Verification items for the finished model (mm, model axes). A direction names the side the tool comes from. Coordinates: 2 decimals unless noted, no trailing zeros. Write each loop counter-clockwise with the first axis right and the second up, starting at its lowest first coordinate (ties: lowest second). Pieces come first, ordered by that corner, then holes. Notation, with made-up numbers: (18, -17.75) -> (54, -17.75) arc R23 cw to (54, -4.75) -> close; hole circle Ø6 at (-14.75, 89.25). An arc over 180 degrees is marked (long way). Use CSV: the item, a comma, the result in double quotes.
```python
from build123d import *

# Parameters (mm, degrees)
F0_R            = 35.76066
F1_DEPTH        = 7.2136
F3_DEPTH        = 7.2146
F3_COPIES_COUNT = 16


# Not quite as in the source:
# - a pattern or mirror of a feature is missing from the dataset's text; its kind, count and spacing are read off the source's solid


with BuildPart() as f1:
    # F0 (on Front) → F1 (new body)
    with BuildSketch(Plane.XZ):
        Circle(F0_R)
    extrude(amount=-F1_DEPTH)

    # F2 (on face) → F3 (cut, through all)
    with BuildSketch(Plane.XZ):
        with BuildLine():
            Line((-4.8164154778, 33.0982711732), (-4.4568878106, 32.3001493474))
            ThreePointArc((-4.4568878106, 32.3001493474), (-3.8441959519, 31.1417538349), (-3.0902142758, 30.0699408338))
            ThreePointArc((-3.0902142758, 30.0699408338), (0, 28.5877), (3.0902142758, 30.0699408338))
            ThreePointArc((3.0902142758, 30.0699408338), (3.8441959519, 31.1417538349), (4.4568878106, 32.3001493474))
            Line((4.4568878106, 32.3001493474), (4.8164154778, 33.0982711732))
            ThreePointArc((4.8164154778, 33.0982711732), (5.4627291736, 34.2224644474), (6.3166306588, 35.198366166))
            ThreePointArc((6.3166306588, 35.198366166), (0, 35.76066), (-6.3166306588, 35.198366166))
            ThreePointArc((-6.3166306588, 35.198366166), (-5.4627291736, 34.2224644474), (-4.8164154778, 33.0982711732))
        make_face()
    f3 = extrude(amount=-F3_DEPTH, mode=Mode.SUBTRACT)

    # F3_copies: F3 ×16 about axis
    f3_copies_axis = Axis((0, 0, 0), (0, 1, 0))
    for i in range(1, F3_COPIES_COUNT):
        add(f3.rotate(f3_copies_axis, i * 360 / F3_COPIES_COUNT), mode=Mode.SUBTRACT)


solid = f1.part
```
1) Set-up check for faces 1 (the cylindrical face through (-18.1, 3.6, -29.5)), 2 (the cylindrical face through (-20.34, 3.56, -28.08)), 3 (the cylindrical face through (15.454, 3.556, 27.289)), 4 (the cylindrical face through (-33.726, 3.556, 8.045)), 5 (the cylindrical face through (34.237, 3.556, 5.473)): record each of +Z, -Z, +X, -X, +Y, -Y from which the full face is reachable in a straight line by a thin tool's end or side.
Return value:
face 1,"-Z, +Y, -Y"
face 2,"-X, +Y, -Y"
face 3,"+Z, +Y, -Y"
face 4,"+Z, -X, +Y, -Y"
face 5,"+X, +Y, -Y"
2) Scan lines: L1, parallel to X at y = 6.25, z = -28; L2, parallel to X at y = 4.25, z = 30; L3, parallel to Z at x = -27, y = 2.25. Record each from-to range of solid material in increasing order.
Return value:
L1,"-20.33 to -16.33, -9.08 to 9.08, 16.33 to 20.33"
L2,"-19.46 to -19.05, -8.41 to -3.03, 3.03 to 8.41, 19.05 to 19.46"
L3,"-20.07 to -15.03, -9.95 to 9.95, 15.03 to 20.07"
3) Cross-section at B-B (x = -10). Record the boundary of the cut face in (y, z).
Return value:
outline,"(0, -26.96) -> (7.21, -26.96) -> (7.21, 26.96) -> (0, 26.96) -> close"
4) Mould release check, pull along Z, two halves, no side actions. Record for faces 6 (the cylindrical face through (28.044, 3.556, 20.333)), 7 (the cylindrical face through (29.5, 3.6, -18.1)), 8 (the cylindrical face through (26.39, 3.56, 10.99)), 9 (the cylindrical face through (8.37, 3.56, -30.22)): released by +Z, released by -Z, zero draft, split by the parting line, or undercut.
Return value:
face 6,"released by +Z"
face 7,"undercut"
face 8,"undercut"
face 9,"released by -Z"
5) Gauge pin test, flat ends, axial feed: pin 1 (1.5 mm diameter, centred on y = 1, z = 5.5, fed in from +X) (3 decimals); pin 2 (4 mm diameter, centred on x = -15, y = 3, fed in from +Z). Record the tip position at first contact, or that the pin passes through.
Return value:
pin 1,"x = 35.135"
pin 2,"z = 28.63"
6) Cross-section at A-A (z = 12.5). Record the boundary of the cut face in (x, y).
Return value:
outline,"(-26.11, 0) -> (26.11, 0) -> (26.11, 7.21) -> (-26.11, 7.21) -> close"
